Autodesk Inventor part; units mm, degrees
ref_plane "Work Plane3" through (-192, -45.5, 9.5) normal (0, 0, 1) x (1, 0, 0)
ref_plane "Work Plane4" through (-192, -45.5, 9.5) normal (0, 0, 1) x (1, 0, 0)
ref_plane "Work Plane5" through (-192, 0, 9.5) normal (0, 0, 1) x (1, 0, 0)
ref_plane "Work Plane1" through (0, -45.5, -2.5) normal (0, 0, -1) x (-1, 0, 0)
ref_plane "Work Plane2" through (0, 0, 0) normal (0, 0, 1) x (1, 0, 0)
sketch "Sketch2" plane through (0, 0, 0) normal (0, 0, 1) x (1, 0, 0)
  line L0 (-191.9993, -42.9912) -> (0.0007, -42.9846) construction
  line L1 (-192.0007, 0.0088) -> (0, 0.0154) construction
  line L2 (-192.0007, 0.0088) -> (-191.9993, -42.9912) construction
  circle A0 centre (-168, -21.4904) radius 7.975 construction
  line L3 (-192.0007, 0.0088) -> (-151.3607, 0.0088)
  line L4 (-151.3607, 0.0088) -> (-151.3607, -42.9898)
  line L5 (-151.3607, -42.9898) -> (-192.0007, -42.9898)
  line L6 (-192.0007, -42.9898) -> (-192.0007, 0.0088)
  circle A1 centre (-168, -21.4904) radius 9.2075
  circle A2 centre (-160, -5.5) radius 2 construction
  circle A3 centre (-160, -37.5) radius 2 construction
  circle A4 centre (-160, -5.5) radius 2.1844
  circle A5 centre (-160, -37.5) radius 2.1844
  circle A6 centre (-184, -37.5) radius 2 construction
  circle A7 centre (-184, -37.5) radius 2.1844
  point P0 (0, 0)
  dimension "d0" = 40.64
  dimension "d1" = 18.415
  dimension "d5" = 4.3688
  dimension "d6" = 4.3688
  dimension "d9" = 4.3688
ref_plane "Work Plane3" through (-192, -45.5, 9.5) normal (0, 0, 1) x (1, 0, 0)
ref_plane "Work Plane4" through (-192, -45.5, 9.5) normal (0, 0, 1) x (1, 0, 0)
ref_plane "Work Plane5" through (-192, 0, 9.5) normal (0, 0, 1) x (1, 0, 0)
extrude "Extrusion3" add sketch "Sketch2" along normal up to surface (9.5 mm away)
sketch "Sketch3" plane through (-192.0007, 0.0088, 9.5) normal (0, 0, 1) x (1, 0, 0)
  circle A0 centre (8.0007, -37.5088) radius 2.1844
  circle A1 centre (32.0007, -37.5088) radius 2.1844
  circle A2 centre (32.0007, -5.5088) radius 2.1844
  point P0 (192.0007, -0.0088)
hole "Hole1" at (-184, -37.5, 9.5) at (-160, -37.5, 9.5) at (-160, -5.5, 9.5) direction (0, 0, -1) diameter 4.3688 end through all counterbore diameter 7.62 counterbore depth 6.985
sketch "Sketch6" plane through (-192.0007, -42.9898, 0) normal (-1, 0, 0) x (0, 0, 1)
  line L0 (4.3851, 29.7217) -> (2.7047, 35.051) construction
  line L1 (0, 42.9986) -> (0, 0)
  line L2 (0, 42.9986) -> (9.5, 12.8685)
  line L3 (9.5, 42.9986) -> (9.5, 0)
  line L4 (0, 42.9986) -> (31.5923, 42.9986) construction
  line L5 (9.5, 12.8685) -> (9.5, 42.9986)
  line L6 (0, 42.9986) -> (9.5, 42.9986)
  line L7 (9.5, 42.9986) -> (0, 42.9986)
  point P0 (0, 42.9898)
  dimension "d23" = 72.5
extrude "Extrusion5" cut sketch "Sketch6" against normal through all
properties part number "BallCasterMountTemp"
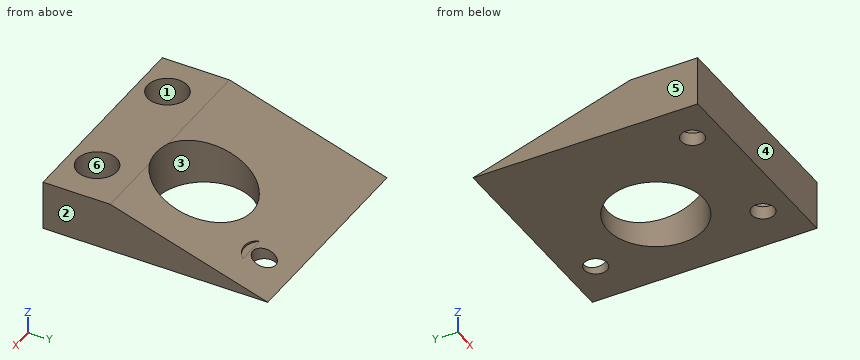
Work out the finished part from the listing and answer in its coordinate system (mm). Face numbers are marked on the shaded views. A direction names the side the tool comes from. Round coordinates to 2 decimals unless told otherwise and drop trailing zeros. Write each loop counter-clockwise with the first axis right and the second up, starting at its lowest first coordinate (ties: lowest second). Pieces come first, ordered by that corner, then holes. Notation, with made-up numbers: (38.5, -40) -> (63.5, -40) arc R16 cw to (63.5, -26) -> close; hole circle Ø9 at (58, 57). An arc over 180 degrees is marked (long way). Write each question's results on one line, items separated by ' | '.
Q1. Flat-ended cylindrical pins translate along their axes: P1, Ø4, axis at x = -182.5, y = -38, coming from the +Z side (3 decimals); P2, Ø5, axis at x = -180, y = -15.5, coming from the +Z side; P3, Ø8, axis at x = -183.5, y = -11, coming from the +Z side. Find the tip coordinate at first contact, or state that the pin passes through.
Data:
P1: z = 2.515 | P2: z = 5.68 | P3: z = 4.73
Q2. Section B-B, the plane x = -176 is taken. Write down the section's boundary in (y, z).
Data:
outline: (-42.99, 0) -> (-26.05, 0) -> (-26.05, 8.22) -> (-30.12, 9.5) -> (-42.99, 9.5) -> close; (-16.93, 0) -> (0.01, 0) -> (-16.93, 5.34) -> close
Q3. Section A-A, the plane y = -37.5 is taken. Write down the section's boundary in (x, z) (3 decimals), then the cut area to 3 significant figures.
Data:
outline: (-192.001, 0) -> (-186.184, 0) -> (-186.184, 2.515) -> (-187.81, 2.515) -> (-187.81, 9.5) -> (-192.001, 9.5) -> close; (-181.816, 0) -> (-162.184, 0) -> (-162.184, 2.515) -> (-163.81, 2.515) -> (-163.81, 9.5) -> (-180.19, 9.5) -> (-180.19, 2.515) -> (-181.816, 2.515) -> close; (-157.816, 0) -> (-151.361, 0) -> (-151.361, 9.5) -> (-156.19, 9.5) -> (-156.19, 2.515) -> (-157.816, 2.515) -> close | area: 258 mm^2
Q4. Straight lines are drawn through the part: line 1 along X through (y, z) = (-37.5, 5); line 2 along Y through (x, z) = (-160, 1.3); line 3 along Y through (x, z) = (-161.5, 8.75). For each, find the intervals that lie inside material, in ascending order. Write a range as [from, to].
Data:
line 1: [-192, -187.81], [-180.19, -163.81], [-156.19, -151.36] | line 2: [-42.99, -39.68], [-35.32, -26.05], [-16.93, -7.68] | line 3: [-42.99, -41], [-34, -28.01]
Q5. Section C-C, the plane y = -5.5 is taken. Write down the section's boundary in (x, z), then the cut area to 3 significant figures.
Data:
outline: (-192, 0) -> (-162.18, 0) -> (-162.18, 1.74) -> (-192, 1.74) -> close; (-157.82, 0) -> (-151.36, 0) -> (-151.36, 1.74) -> (-157.82, 1.74) -> close | area: 63.0 mm^2
Q6. Determine the mould class of the marked faces 1, 2, 3 and 4 for opening direction Y: released by +Y, released by -Y, zero draft, split by the parting line, or undercut.
Data:
face 1: undercut | face 2: zero draft | face 3: undercut | face 4: released by -Y
Q7. Which of the six approach directions +Z, -Z, +X, -X, +Y, -Y give full straight-line access (tool end or side, diameter ignored) to the marked faces 5 and 6?
Data:
face 5: +Z, -Z, -X, +Y, -Y | face 6: +Z
Q8. Section D-D, the plane z = 1 is taken. Write down the section's boundary in (x, y) (1 decimal).
Data:
outline: (-192, -43) -> (-151.4, -43) -> (-151.4, -3.2) -> (-192, -3.2) -> close; hole circle Ø4.4 at (-184, -37.5); hole circle Ø18.4 at (-168, -21.5); hole circle Ø4.4 at (-160, -37.5); hole circle Ø4.4 at (-160, -5.5)
